Geometry check sheet. Reference: the model listing, model coordinates, mm. Face numbers are marked on the shaded views. A direction names the side the tool comes from. Give positions to 0.01 mm unless a question says otherwise; leave off trailing zeros. Order: outer loops, then holes, each group sorted by start corner. A loop starts at its lowest first (then second) coordinate and runs counter-clockwise, first axis right, second up.
```python
from build123d import *

# Parameters (mm, degrees)
F1_DEPTH = 10.31875
F2_R     = 3.90906
F3_DEPTH = 25.4
F4_DEPTH = 25.4
F6_R     = 7.14375
F7_DEPTH = 2.3495
F8_R     = 6.38175
F9_DEPTH = 1.5875
F10_R    = 0.4064


# Not quite as in the source:
# - a fillet or chamfer that OpenCascade refuses, or shapes differently, is made with other operations: its cross-section is extruded or revolved along the edge and cut away or added


with BuildPart() as f1:
    # F0 (on Top) → F1 (new body, symmetric)
    with BuildSketch(Plane.XY):
        with BuildLine():
            Line((0, 20.6466445854), (-11.58875, 20.6466445854))
            ThreePointArc((-11.58875, 20.6466445854), (-17.1096965819, 19.861848606), (-22.19325, 17.5696355848))
            Line((-22.19325, 17.5696355848), (-22.19325, -17.5696355848))
            ThreePointArc((-22.19325, -17.5696355848), (-17.1096965819, -19.861848606), (-11.58875, -20.6466445854))
            Line((-11.58875, -20.6466445854), (0, -20.6466445854))
            Line((0, -20.6466445854), (11.58875, -20.6466445854))
            ThreePointArc((11.58875, -20.6466445854), (17.1096965819, -19.861848606), (22.19325, -17.5696355848))
            Line((22.19325, -17.5696355848), (22.19325, 17.5696355848))
            ThreePointArc((22.19325, 17.5696355848), (17.1096965819, 19.861848606), (11.58875, 20.6466445854))
            Line((11.58875, 20.6466445854), (0, 20.6466445854))
        make_face()
        with BuildLine():
            ThreePointArc((11.58875, 19.8846445854), (16.6970877606, 19.1869573913), (21.43125, 17.145))
            Line((21.43125, 17.145), (21.43125, -17.145))
            ThreePointArc((21.43125, -17.145), (16.6970877606, -19.1869573913), (11.58875, -19.8846445854))
            Line((11.58875, -19.8846445854), (0, -19.8846445854))
            Line((0, -19.8846445854), (-11.58875, -19.8846445854))
            ThreePointArc((-11.58875, -19.8846445854), (-16.6970877606, -19.1869573913), (-21.43125, -17.145))
            Line((-21.43125, -17.145), (-21.43125, 17.145))
            ThreePointArc((-21.43125, 17.145), (-16.6970877606, 19.1869573913), (-11.58875, 19.8846445854))
            Line((-11.58875, 19.8846445854), (0, 19.8846445854))
            Line((0, 19.8846445854), (11.58875, 19.8846445854))
        make_face(mode=Mode.SUBTRACT)
    extrude(amount=F1_DEPTH, both=True)

    # F2 (on face) → F3 (cut)
    with BuildSketch(Plane.YZ.offset(22.19325)):
        with BuildLine():
            ThreePointArc((0.396875, -6.3375855209), (4.6283180665, -4.3475478002), (6.35, 0))
            ThreePointArc((6.35, 0), (4.6283180665, 4.3475478002), (0.396875, 6.3375855209))
            Line((0.396875, 6.3375855209), (0.396875, -6.3375855209))
        make_face()
        with BuildLine():
            Line((0.396875, -6.3375855209), (0.396875, 6.3375855209))
            ThreePointArc((0.396875, 6.3375855209), (0, 6.35), (-0.396875, 6.3375855209))
            Line((-0.396875, 6.3375855209), (-0.396875, -6.3375855209))
            ThreePointArc((-0.396875, -6.3375855209), (0, -6.35), (0.396875, -6.3375855209))
        make_face()
        with BuildLine():
            ThreePointArc((-0.396875, 6.3375855209), (0, 6.35), (0.396875, 6.3375855209))
            Line((0.396875, 6.3375855209), (0.396875, 16.235569492))
            Line((0.396875, 16.235569492), (-0.396875, 16.235569492))
            Line((-0.396875, 16.235569492), (-0.396875, 6.3375855209))
        make_face()
        with BuildLine():
            Line((0.396875, -16.235569492), (0.396875, -6.3375855209))
            ThreePointArc((0.396875, -6.3375855209), (0, -6.35), (-0.396875, -6.3375855209))
            Line((-0.396875, -6.3375855209), (-0.396875, -16.235569492))
            Line((-0.396875, -16.235569492), (0.396875, -16.235569492))
        make_face()
        with BuildLine():
            Line((-0.396875, -6.3375855209), (-0.396875, 6.3375855209))
            ThreePointArc((-0.396875, 6.3375855209), (-6.35, 0), (-0.396875, -6.3375855209))
        make_face()
        with Locations((-11.9634, 0)):
            Circle(F2_R)
        with Locations((11.9634, 0)):
            Circle(F2_R)
    extrude(amount=-F3_DEPTH, mode=Mode.SUBTRACT)

    # F2 (on face) → F4 (cut)
    with BuildSketch(Plane.YZ.offset(22.19325)):
        with BuildLine():
            ThreePointArc((0.396875, -6.3375855209), (4.6283180665, -4.3475478002), (6.35, 0))
            ThreePointArc((6.35, 0), (4.6283180665, 4.3475478002), (0.396875, 6.3375855209))
            Line((0.396875, 6.3375855209), (0.396875, -6.3375855209))
        make_face()
        with BuildLine():
            Line((0.396875, -6.3375855209), (0.396875, 6.3375855209))
            ThreePointArc((0.396875, 6.3375855209), (0, 6.35), (-0.396875, 6.3375855209))
            Line((-0.396875, 6.3375855209), (-0.396875, -6.3375855209))
            ThreePointArc((-0.396875, -6.3375855209), (0, -6.35), (0.396875, -6.3375855209))
        make_face()
        with BuildLine():
            ThreePointArc((-0.396875, 6.3375855209), (0, 6.35), (0.396875, 6.3375855209))
            Line((0.396875, 6.3375855209), (0.396875, 16.235569492))
            Line((0.396875, 16.235569492), (-0.396875, 16.235569492))
            Line((-0.396875, 16.235569492), (-0.396875, 6.3375855209))
        make_face()
        with BuildLine():
            Line((0.396875, -16.235569492), (0.396875, -6.3375855209))
            ThreePointArc((0.396875, -6.3375855209), (0, -6.35), (-0.396875, -6.3375855209))
            Line((-0.396875, -6.3375855209), (-0.396875, -16.235569492))
            Line((-0.396875, -16.235569492), (0.396875, -16.235569492))
        make_face()
        with BuildLine():
            Line((-0.396875, -6.3375855209), (-0.396875, 6.3375855209))
            ThreePointArc((-0.396875, 6.3375855209), (-6.35, 0), (-0.396875, -6.3375855209))
        make_face()
        with Locations((-11.9634, 0)):
            Circle(F2_R)
        with Locations((11.9634, 0)):
            Circle(F2_R)
    extrude(amount=-F4_DEPTH, mode=Mode.SUBTRACT)

    # F5: chamfer of 0.762 x 0.8765807263 on 2 edges, made by hand

    # F5_s1 → F5_t2 (revolve, cut)
    with BuildSketch(Plane.XY):
        Polygon((22.19325, -7.1777592737), (21.43125, -8.05434), (22.19325, -8.05434), align=None)
    revolve(axis=Axis((22.19325, -11.9634, 0), (1, 0, 0)), mode=Mode.SUBTRACT)

    # F5_s3 → F5_t4 (revolve, cut)
    with BuildSketch(Plane.XY):
        Polygon((22.19325, 16.63446), (21.3166692737, 15.87246), (22.19325, 15.87246), align=None)
    revolve(axis=Axis((22.19325, 11.9634, 0), (1, 0, 0)), mode=Mode.SUBTRACT)

    # F6 (on face) → F7 (join)
    with BuildSketch(Plane(origin=(-22.19325, 0, 0), x_dir=(0, -1, 0), z_dir=(-1, 0, 0))):
        Circle(F6_R)
    extrude(amount=-F7_DEPTH)

    # F8 (on face) → F9 (cut)
    with BuildSketch(Plane(origin=(-22.19325, 0, 0), x_dir=(0, -1, 0), z_dir=(-1, 0, 0))):
        Circle(F8_R)
    extrude(amount=-F9_DEPTH, mode=Mode.SUBTRACT)

    # F10
    f10_edges = [f1.edges().sort_by_distance(p)[0] for p in [
        (-22.19325, 6.38175, 0),
        (-20.60575, 6.38175, 0),
        (-19.84375, 7.14375, 0),
    ]]
    fillet(f10_edges, radius=F10_R)


solid = f1.part
```
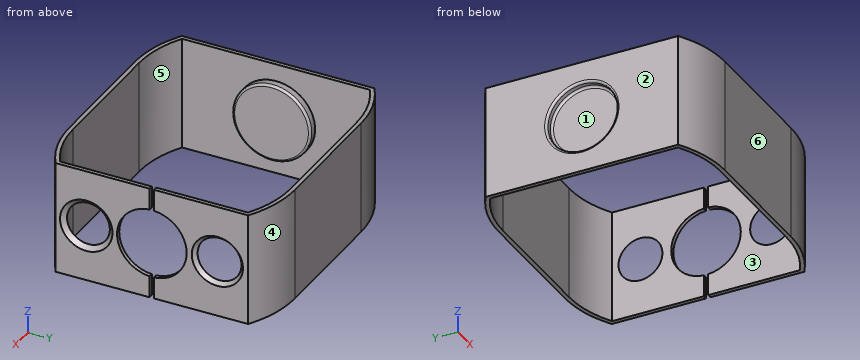
Q1. Gauge pin test, flat ends, axial feed: P1, Ø6.5, axis at y = -2.5, z = 2, coming from the +X side; P2, Ø11.5, axis at y = 0, z = 0, coming from the -X side. Record the tip position at first contact, or that the pin passes through.
Q2. Cross-section at A-A, the plane x = 5. Record the boundary of the cut face in (y, z), and give its area (3 significant figures).
Q3. Access from +Z, -Z, +X, -X, +Y, -Y to the whole of each face (thin tool, end or side, straight path). Record for the marked faces 1, 2 and 3.
Q4. Thickness scan on L1, parallel to X at y = -14, z = 8; L2, parallel to Y at x = 3, z = 4.5; L3, parallel to Z at x = -21.3, y = 0. Record the ranges inside material, lowest first.
Q5. Cross-section at B-B, the plane z = 7.75. Record the boundary of the cut face in (x, y) (3 decimals).
Q6. Cross-section at C-C, the plane z = -3.25. Give the number of separate pieces and of enclosed holes in the cut face, and give its area (3 significant figures).
Q7. Release check for a two-part mould opening along X. For the marked faces 4, 5 and 6 record: pulls with the +X half, pulls with the -X half, needs draft (parallel to the pull), parting line crosses it, or undercut.
Answers follow:
1. P1: stops at x = 22.19
1. P2: stops at x = -20.61
2. outline: (-20.65, -10.32) - (-19.88, -10.32) - (-19.88, 10.32) - (-20.65, 10.32) - close; (19.88, -10.32) - (20.65, -10.32) - (20.65, 10.32) - (19.88, 10.32) - close
2. area: 31.5 mm2
3. face 1: -X
3. face 2: +Z, -Z, -X, +Y, -Y
3. face 3: +Z, -Z
4. L1: x = -22.19 to -21.43, 21.43 to 22.19
4. L2: y = -20.65 to -19.88, 19.88 to 20.65
4. L3: z = -7.14 to -6.38, 6.38 to 7.14
5. outline: (-22.193, -17.57) arc R19.812 ccw to (-11.589, -20.647) - (11.589, -20.647) arc R19.812 ccw to (22.193, -17.57) - (22.193, -0.397) - (21.431, -0.397) - (21.431, -17.145) arc R19.05 cw to (11.589, -19.885) - (-11.589, -19.885) arc R19.05 cw to (-21.431, -17.145) - (-21.431, 17.145) arc R19.05 cw to (-11.589, 19.885) - (11.589, 19.885) arc R19.05 cw to (21.431, 17.145) - (21.431, 0.397) - (22.193, 0.397) - (22.193, 17.57) arc R19.812 ccw to (11.589, 20.647) - (-11.589, 20.647) arc R19.812 ccw to (-22.193, 17.57) - close
6. separate pieces: 3
6. enclosed holes: 0
6. area: 107 mm2
7. face 4: pulls with the +X half
7. face 5: undercut
7. face 6: needs draft
